from build123d import *

# Parameters (mm, degrees)
F1_DEPTH = 10.922
F3_DEPTH = 13.462
F5_DEPTH = 9.906


with BuildPart() as f1:
    # F0 (on Right) → F1 (new body)
    with BuildSketch(Plane.YZ):
        Polygon((0, 55.701409), (-46.533596, 55.701409), (-46.533596, -40.143907), (0, -40.143907), (0, -26.808906), align=None)
        Polygon((17.918905, -26.808906), (0, -26.808906), (0, -40.143907), (0, -40.421717), (17.918905, -40.421717), align=None)
    extrude(amount=F1_DEPTH)

    # F2 (on face) → F3 (join)
    with BuildSketch(Plane.YZ.offset(10.922)):
        Polygon((0, 55.701409), (-10.959693, 55.701409), (-10.959693, -40.143907), (0, -40.143907), (0, -26.808906), align=None)
        Polygon((17.918905, -26.808906), (0, -26.808906), (0, -40.143907), (0, -40.421717), (17.918905, -40.421717), align=None)
    extrude(amount=F3_DEPTH)

    # F4 (on face) → F5 (join)
    with BuildSketch(Plane.YZ.offset(24.384)):
        Polygon((35.362165, 55.701409), (0, 55.701409), (0, -26.808906), (17.918905, -26.808906), (17.918905, -40.421717), (35.362165, -40.421717), align=None)
        Polygon((0, 55.701409), (-10.959693, 55.701409), (-10.959693, -40.143907), (0, -40.143907), (0, -40.421717), (17.918905, -40.421717), (17.918905, -26.808906), (0, -26.808906), align=None)
    extrude(amount=F5_DEPTH)


solid = f1.part
Part model, mm, in its own coordinate system. A direction names the side the tool comes from. Coordinates: 2 decimals unless noted, no trailing zeros. Loops run counter-clockwise (first coordinate to the right, second up) from the corner with the lowest first, then second, coordinate; pieces in that order, holes last. Notation, with made-up numbers: (22, -14) - (58, -14) arc R24 ccw to (58, 18) - close; hole circle Ø5 at (65.25, -26). An arc over 180 degrees is marked (long way). Write each question's results on one line, items separated by ' | '. Start each with the question number.
Q1. Probe line 1 along Z through (x, y) = (7, -24.5); line 2 along X through (y, z) = (-28, 50.5); line 3 along Y through (x, z) = (13, 6.5). List the from-to ranges inside material, lowest first.
Q2. Which spindle directions (+Z, -Z, +X, -X, +Y, -Y) get a long thin tool onto all of the face, cutting with end or side? Do faces 1 (the flat face through (17, -5, 55.701)), 2 (the flat face through (22, -10.96, 8)), 3 (the flat face through (12, 9, -26.809)), 4 (the flat face through (12, 17.919, -34)), 5 (the flat face through (9, -18, -40.144)). Say none if no direction does.
Q3. Slice it at C-C on y = 13. Give the cut face in (x, z), and give its area (3 significant figures).
Q4. Drop flat-ended pins along their axis: pin 1 Ø10.5 at (y, z) = (-37.5, 25.5) entering from +X; pin 2 Ø2 at (x, z) = (14.5, -3) entering from +Y; pin 3 Ø4 at (x, z) = (23, 42) entering from -Y. Give the stop position or say it passes through.
Q5. Slice it at D-D on y = 29.5. Give the cut face in (x, z).
Q6. Slice it at A-A on z = -17. Give the cut face in (x, y).
Q7. Slice it at B-B on x = 5. Give the cut face in (y, z), and give its area (3 significant figures).
Answer:
1) line 1: z = -40.14 to 55.7 | line 2: x = 0 to 10.92 | line 3: y = -10.96 to 0
2) face 1: +Z, +X, -X, +Y, -Y | face 2: +Z, -Z, +X, -Y | face 3: +Z, -X, +Y | face 4: +Z, -Z, -X, +Y | face 5: -Z, +X, -X, -Y
3) outline: (0, -40.42) - (34.29, -40.42) - (34.29, 55.7) - (24.38, 55.7) - (24.38, -26.81) - (0, -26.81) - close | area: 1,280 mm2
4) pin 1: stops at x = 10.92 | pin 2: stops at y = 0 | pin 3: stops at y = -10.96
5) outline: (24.38, -40.42) - (34.29, -40.42) - (34.29, 55.7) - (24.38, 55.7) - close
6) outline: (0, -46.53) - (10.92, -46.53) - (10.92, -10.96) - (34.29, -10.96) - (34.29, 35.36) - (24.38, 35.36) - (24.38, 0) - (0, 0) - close
7) outline: (-46.53, -40.14) - (0, -40.14) - (0, -40.42) - (17.92, -40.42) - (17.92, -26.81) - (0, -26.81) - (0, 55.7) - (-46.53, 55.7) - close | area: 4,700 mm2
